Drawing for the job (mm, zero at the part's lowest x, y, z). A direction names the side the tool comes from. Give positions to 0.01 mm unless a question says otherwise; leave off trailing zeros. Write each loop counter-clockwise with the first axis right and the second up, starting at its lowest first coordinate (ties: lowest second). Pieces come first, ordered by that corner, then holes. Notation, with made-up numbers: M 88,58 L 112,58 A17 cw 112,81 Z; hole C 6,39.5 d1. An arc over 180 degrees is marked long. Use a Markdown table: item, result. Add a question column.
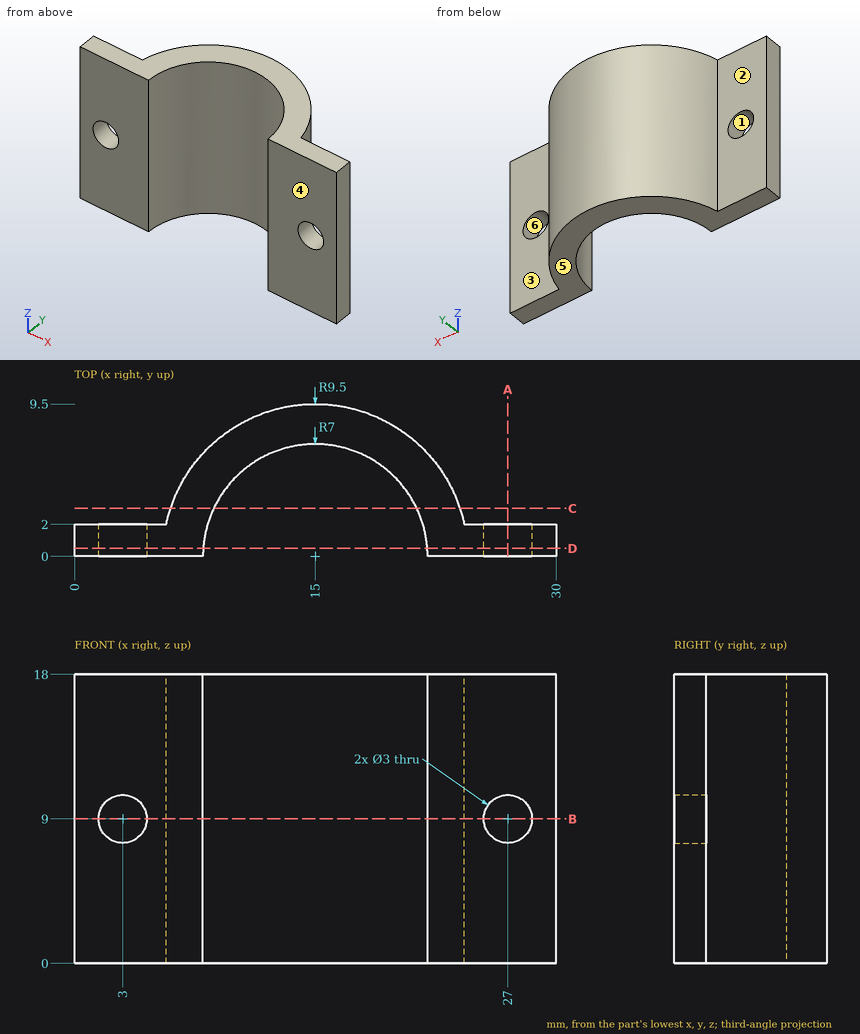
1. Cut at B-B (z = 9). Write the cut outline in (x, y).
2. Mould opens along Z. For the marked faces 4, 5 and 6 say: released by +Z, released by -Z, zero draft, split by the parting line, or undercut.
3. Tool access for the marked faces 1, 2 and 3: list every direction of +Z, -Z, +X, -X, +Y, -Y with a clear straight run to the whole face (end or side of a thin tool).
4. Cut at A-A (x = 27). Write the cut outline in (y, z).
5. Cut at D-D (y = 0.5). Write the cut outline in (x, z), then the cut area to 3 significant figures.
6. Flat gauge pins, fed straight in: pin 1 (3 mm diameter, centred on x = 25, z = 8.5, fed in from +Y); pin 2 (3.5 mm diameter, centred on x = 3, z = 9, fed in from +Y); pin 3 (1 mm diameter, centred on y = 4.5, z = 5.5, fed in from -X). Where does each tip first touch, or does it go through?
7. Cut at C-C (y = 3). Write the cut outline in (x, z).
8. Drill centre lines: probe 1 along Z at (x, y) = (3, 1.2); probe 2 along X at (y, z) = (0.95, 9); probe 3 along Y at (x, z) = (3.5, 11). Where is each one in solid material? Low to high. Write a range as [from, to].
A:
| question | item | result |
|---|---|---|
| 1 | outline | M 0,0 L 1.5,0 L 1.5,2 L 0,2 Z; M 4.5,0 L 8,0 A7 cw 22,0 L 25.5,0 L 25.5,2 L 24.29,2 A9.5 ccw 5.71,2 L 4.5,2 Z; M 28.5,0 L 30,0 L 30,2 L 28.5,2 Z |
| 2 | face 4 | zero draft |
| 2 | face 5 | released by -Z |
| 2 | face 6 | undercut |
| 3 | face 1 | +Y, -Y |
| 3 | face 2 | +Z, -Z, -X, +Y |
| 3 | face 3 | +Z, -Z, +X, +Y |
| 4 | outline | M 0,0 L 2,0 L 2,7.5 L 0,7.5 Z; M 0,10.5 L 2,10.5 L 2,18 L 0,18 Z |
| 5 | outline | M 0,0 L 8.02,0 L 8.02,18 L 0,18 Z; M 21.98,0 L 30,0 L 30,18 L 21.98,18 Z; hole C 3,9 d3; hole C 27,9 d3 |
| 5 | area | 275 mm² |
| 6 | pin 1 | stops at y = 4.24 |
| 6 | pin 2 | stops at y = 2 |
| 6 | pin 3 | stops at x = 6.38 |
| 7 | outline | M 5.99,0 L 8.68,0 L 8.68,18 L 5.99,18 Z; M 21.32,0 L 24.01,0 L 24.01,18 L 21.32,18 Z |
| 8 | probe 1 | z = [0, 7.5], [10.5, 18] |
| 8 | probe 2 | x = [0, 1.5], [4.5, 8.06], [21.94, 25.5], [28.5, 30] |
| 8 | probe 3 | y = [0, 2] |
